Geometry: final body of the model. Coordinates: model frame, mm. Face numbers are marked on the shaded views. A direction names the side the tool comes from. Coordinates: 2 decimals unless noted, no trailing zeros. Write each loop counter-clockwise with the first axis right and the second up, starting at its lowest first coordinate (ties: lowest second). Pieces come first, ordered by that corner, then holes. Notation, with made-up numbers: (-28, 10.25) - (-15, 10.25) arc R17 cw to (-15, 20.25) - close; hole circle Ø8 at (37, -4.75). An arc over 180 degrees is marked (long way). Answer as a JSON object with one key per item and string values. Group by question number.
Item 1: Line query: line 1 along Y through (x, z) = (7.75, 1.2); line 2 along Z through (x, y) = (-6.5, -15); line 3 along Y through (x, z) = (-17, -31). Output: solid intervals per line, ascending. Write a range as from..to.
Item 2: Section D-D on x = 15. Return loops of the section in (y, z), and give its area (3 significant figures).
Item 3: Set-up query: the marked faces 1 and 2. Return all of +Z, -Z, +X, -X, +Y, -Y with unobstructed straight access to the full face (end or side cutting, diameter ignored); none if empty.
Item 4: Section A-A on y = -2.5. Return loops of the section in (x, z), and give its area (3 significant figures).
Item 5: Section B-B on x = 7.5. Return loops of the section in (y, z), and give its area (3 significant figures).
Item 6: Section C-C on z = -36. Return loops of the section in (x, y).
Item 7: First-contact query: pin 1 Ø5 at (x, y) = (7.75, 13.42) entering from -Z; pin 2 Ø2 at (x, z) = (14.5, -18.5) entering from +Y; pin 3 Ø2.5 at (x, y) = (-7.75, -13.42) entering from -Z. Flat tips, straight axial feed; report the tip coordinate or a pass-through.
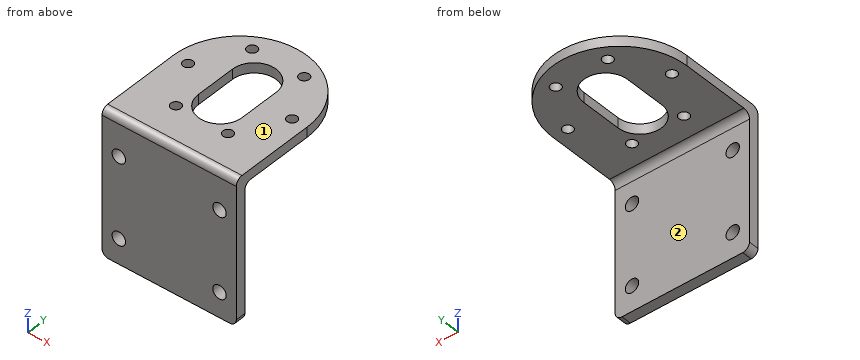
```python
from build123d import *

# Parameters (mm, degrees)
SKETCH_1_R      = 1.5
EXTRUDE_1_DEPTH = 3
SKETCH_2_R      = 2
EXTRUDE_2_DEPTH = 3
FILLET_1_R      = 2


with BuildPart() as part:
    # 草图1 → 凸台-拉伸1 (new body)
    with BuildSketch(Plane.XY):
        with BuildLine():
            Line((-20, 0), (-20, -25))
            Line((-20, -25), (20, -25))
            Line((20, -25), (20, 0))
            ThreePointArc((20, 0), (0, 20), (-20, 0))
        make_face()
        with Locations((7.75, 13.423393759)):
            Circle(SKETCH_1_R, mode=Mode.SUBTRACT)
        with Locations((15.5, 0)):
            Circle(SKETCH_1_R, mode=Mode.SUBTRACT)
        with Locations((7.75, -13.423393759)):
            Circle(SKETCH_1_R, mode=Mode.SUBTRACT)
        with Locations((-7.75, -13.423393759)):
            Circle(SKETCH_1_R, mode=Mode.SUBTRACT)
        with Locations((-15.5, 0)):
            Circle(SKETCH_1_R, mode=Mode.SUBTRACT)
        with Locations((-7.75, 13.423393759)):
            Circle(SKETCH_1_R, mode=Mode.SUBTRACT)
        with BuildLine():
            Line((6.5, 5), (6.5, -7))
            ThreePointArc((6.5, -7), (0, -13.5), (-6.5, -7))
            Line((-6.5, -7), (-6.5, 5))
            ThreePointArc((-6.5, 5), (0, 11.5), (6.5, 5))
        make_face(mode=Mode.SUBTRACT)
    extrude(amount=EXTRUDE_1_DEPTH)

    # 草图2 → 凸台-拉伸2 (add)
    with BuildSketch(Plane.XZ.offset(25)):
        with BuildLine():
            Line((20, 0), (-20, 0))
            Line((-20, 0), (-20, -38))
            ThreePointArc((-20, -38), (-19.414213562, -39.414213562), (-18, -40))
            Line((-18, -40), (18, -40))
            ThreePointArc((18, -40), (19.414213562, -39.414213562), (20, -38))
            Line((20, -38), (20, 0))
        make_face()
        with Locations(Location((-15, -32.5, 0), (0, 0, 270))):
            Circle(SKETCH_2_R, mode=Mode.SUBTRACT)
        with Locations(Location((-15, -8.5, 0), (0, 0, 90))):
            Circle(SKETCH_2_R, mode=Mode.SUBTRACT)
        with Locations(Location((15, -32.5, 0), (0, 0, 90))):
            Circle(SKETCH_2_R, mode=Mode.SUBTRACT)
        with Locations(Location((15, -8.5, 0), (0, 0, 270))):
            Circle(SKETCH_2_R, mode=Mode.SUBTRACT)
    extrude(amount=-EXTRUDE_2_DEPTH)

    # 圆角1
    fillet_1_edges = [part.edges().sort_by_distance(p)[0] for p in [
        (0, -25, 3),
        (0, -22, 0),
    ]]
    fillet(fillet_1_edges, radius=FILLET_1_R)


solid = part.part
```
Checks:
{
 "1": {"line 1": "-24.99..-14.92, -11.92..11.92, 14.92..18.44", "line 2": "0..3", "line 3": "-25..-22"},
 "2": {"outline": "(-25, -40) - (-22, -40) - (-22, -34.5) - (-25, -34.5) - close; (-25, -30.5) - (-22, -30.5) - (-22, -10.5) - (-25, -10.5) - close; (-25, -6.5) - (-22, -6.5) - (-22, -2) arc R2 cw to (-20, 0) - (-1.41, 0) - (-1.41, 3) - (-23, 3) arc R2 ccw to (-25, 1) - close; (1.41, 0) - (13.23, 0) - (13.23, 3) - (1.41, 3) - close", "area": "202 mm^2"},
 "3": {"face 1": "+Z, +X, -X, +Y, -Y", "face 2": "-Z, +X, -X, +Y"},
 "4": {"outline": "(-20, 0) - (-6.5, 0) - (-6.5, 3) - (-20, 3) - close; (6.5, 0) - (20, 0) - (20, 3) - (6.5, 3) - close", "area": "81.0 mm^2"},
 "5": {"outline": "(-25, -40) - (-22, -40) - (-22, -2) arc R2 cw to (-20, 0) - (-14.9, 0) - (-14.9, 3) - (-23, 3) arc R2 ccw to (-25, 1) - close; (-11.94, 0) - (11.94, 0) - (11.94, 3) - (-11.94, 3) - close; (14.9, 0) - (18.54, 0) - (18.54, 3) - (14.9, 3) - close", "area": "233 mm^2"},
 "6": {"outline": "(-20, -25) - (20, -25) - (20, -22) - (-20, -22) - close"},
 "7": {"pin 1": "z = 0", "pin 2": "y = -22", "pin 3": "through"}
}
